from build123d import *

# Parameters (mm, degrees)
F0_W     = 73
F0_H     = 48
F1_DEPTH = 4
F0_W_2   = 79
F0_H_2   = 54
F2_DEPTH = 25
F3_W     = 2
F3_H     = 12
F4_DEPTH = 54
F5_W     = 20
F5_H     = 12
F6_DEPTH = 8
F7_W     = 3.5
F7_H     = 8
F8_DEPTH = 80
F9_R     = 3
F10_R    = 1


with BuildPart() as f1:
    # F0 (on Top) → F1 (new body)
    with BuildSketch(Plane.XY):
        Rectangle(F0_W, F0_H)
    extrude(amount=F1_DEPTH)

    # F0 (on Top) → F2 (join)
    with BuildSketch(Plane.XY):
        Rectangle(F0_W_2, F0_H_2)
        Rectangle(F0_W, F0_H, mode=Mode.SUBTRACT)
    extrude(amount=F2_DEPTH)

    # F3 (on face) → F4 (join)
    with BuildSketch(Plane.XZ.offset(27)):
        with Locations((40.5, 19)):
            Rectangle(F3_W, F3_H)
        Polygon((39.5, 13), (39.5, 0), (41.5, 13), align=None)
        with Locations((-40.5, 19)):
            Rectangle(F3_W, F3_H)
        Polygon((-41.5, 13), (-39.5, 0), (-39.5, 13), align=None)
    extrude(amount=-F4_DEPTH)

    # F5 (on face) → F6 (join)
    with BuildSketch(Plane(origin=(0, 27, 0), x_dir=(-1, 0, 0), z_dir=(0, 1, 0))):
        with Locations((-25.5, 19)):
            Rectangle(F5_W, F5_H)
        with Locations((25.5, 19)):
            Rectangle(F5_W, F5_H)
    extrude(amount=F6_DEPTH)

    # F7 (on face) → F8 (cut)
    with BuildSketch(Plane(origin=(-35.5, 0, 0), x_dir=(0, -1, 0), z_dir=(-1, 0, 0))):
        with Locations((-28.75, 17)):
            Rectangle(F7_W, F7_H)
    extrude(amount=-F8_DEPTH, mode=Mode.SUBTRACT)

    # F9
    f9_edges = [f1.edges().sort_by_distance(p)[0] for p in [
        (0, -24, 4),
        (36.5, 0, 4),
        (0, 24, 4),
        (-36.5, 0, 4),
    ]]
    fillet(f9_edges, radius=F9_R)

    # F10
    f10_edges = [f1.edges().sort_by_distance(p)[0] for p in [
        (0, -27, 25),
        (41.5, 0, 25),
        (38.5, 27, 25),
        (35.5, 31, 25),
        (25.5, 35, 25),
        (15.5, 31, 25),
        (0, 27, 25),
        (-15.5, 31, 25),
        (-25.5, 35, 25),
        (-35.5, 31, 25),
        (-38.5, 27, 25),
        (-41.5, 0, 25),
        (36.5, 0, 25),
        (0, -24, 25),
        (-36.5, 0, 25),
        (0, 24, 25),
        (0, -27, 0),
        (39.5, 0, 0),
        (0, 27, 0),
        (-39.5, 0, 0),
        (-40.5, -27, 6.5),
        (-41.5, -27, 19),
        (41.5, -27, 19),
        (40.5, -27, 6.5),
        (41.5, 0, 13),
        (40.5, 27, 6.5),
        (41.5, 27, 19),
        (-41.5, 0, 13),
        (-40.5, 27, 6.5),
        (-41.5, 27, 19),
        (-15.5, 35, 19),
        (-25.5, 35, 13),
        (-35.5, 35, 19),
        (35.5, 35, 19),
        (25.5, 35, 13),
        (15.5, 35, 19),
        (25.5, 30.5, 13),
        (15.5, 32.75, 13),
        (35.5, 32.75, 13),
        (-25.5, 30.5, 13),
        (-35.5, 32.75, 13),
        (-15.5, 32.75, 13),
        (-15.5, 27, 23),
        (-15.5, 28.75, 21),
        (-15.5, 30.5, 17),
        (35.5, 27, 23),
        (35.5, 28.75, 21),
        (35.5, 30.5, 17),
        (15.5, 30.5, 17),
        (15.5, 28.75, 21),
        (15.5, 27, 23),
        (-35.5, 30.5, 17),
        (-35.5, 28.75, 21),
        (-35.5, 27, 23),
        (25.5, 27, 21),
        (-25.5, 27, 21),
    ]]
    fillet(f10_edges, radius=F10_R)


solid = f1.part
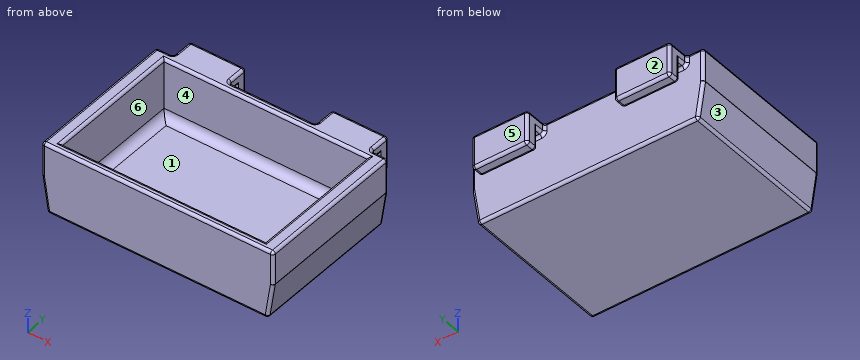
Geometry check sheet. Reference: the model listing, model coordinates, mm. Face numbers are marked on the shaded views. A direction names the side the tool comes from. Give positions to 0.01 mm unless a question says otherwise; leave off trailing zeros. Order: outer loops, then holes, each group sorted by start corner. A loop starts at its lowest first (then second) coordinate and runs counter-clockwise, first axis right, second up.
1) Gauge pin test, flat ends, axial feed: pin 1 (3 mm diameter, centred on y = 32, z = 20, fed in from +X); pin 2 (3 mm diameter, centred on x = -29, y = 29.5, fed in from -Z); pin 3 (5 mm diameter, centred on y = 32, z = 18, fed in from -X). Record the tip position at first contact, or that the pin passes through.
Results are:
pin 1: stops at x = 35.5
pin 2: stops at z = 13.13
pin 3: stops at x = -35.5
2) Cross-section at A-A (z = 17.25). Record the boundary of the cut face in (x, y).
Results are:
outline: (-41.5, -26) arc R1 ccw to (-40.5, -27) - (40.5, -27) arc R1 ccw to (41.5, -26) - (41.5, 26) arc R1 ccw to (40.5, 27) - (-40.5, 27) arc R1 ccw to (-41.5, 26) - close; (-35.5, 31.5) arc R1 ccw to (-34.5, 30.5) - (-16.5, 30.5) arc R1 ccw to (-15.5, 31.5) - (-15.5, 34) arc R1 ccw to (-16.5, 35) - (-34.5, 35) arc R1 ccw to (-35.5, 34) - close; (15.5, 31.5) arc R1 ccw to (16.5, 30.5) - (34.5, 30.5) arc R1 ccw to (35.5, 31.5) - (35.5, 34) arc R1 ccw to (34.5, 35) - (16.5, 35) arc R1 ccw to (15.5, 34) - close; hole (-36.5, -24) - (36.5, -24) - (36.5, 24) - (-36.5, 24) - close
3) Draft check along X on the marked faces 1, 2, 3 and 4. Enter one of: released by +X, released by -X, zero draft, split by the parting line, or undercut.
Results are:
face 1: undercut
face 2: zero draft
face 3: released by -X
face 4: undercut
4) Material ranges on probe 1 along Y at (x, z) = (-34.5, 17); probe 2 along Y at (x, z) = (36, 11.5); probe 3 along Z at (x, y) = (-6, 21), recorded low to high.
Results are:
probe 1: y = -27 to -24, 24 to 27, 30.5 to 35
probe 2: y = -27 to -24, 24 to 27
probe 3: z = 0 to 4
5) Cross-section at B-B (z = 23). Record the boundary of the cut face in (x, y).
Results are:
outline: (-41.5, -26) arc R1 ccw to (-40.5, -27) - (40.5, -27) arc R1 ccw to (41.5, -26) - (41.5, 26) arc R1 ccw to (40.5, 27) - (36.5, 27) arc R1 cw to (35.5, 28) - (35.5, 34) arc R1 ccw to (34.5, 35) - (16.5, 35) arc R1 ccw to (15.5, 34) - (15.5, 28) arc R1 cw to (14.5, 27) - (-14.5, 27) arc R1 cw to (-15.5, 28) - (-15.5, 34) arc R1 ccw to (-16.5, 35) - (-34.5, 35) arc R1 ccw to (-35.5, 34) - (-35.5, 28) arc R1 cw to (-36.5, 27) - (-40.5, 27) arc R1 ccw to (-41.5, 26) - close; hole (-36.5, -24) - (36.5, -24) - (36.5, 24) - (-36.5, 24) - close
6) Cross-section at D-D (y = -19.5). Record the boundary of the cut face in (x, z).
Results are:
outline: (-41.5, 13.08) arc R1 ccw to (-41.49, 12.92) - (-39.63, 0.85) arc R1 ccw to (-38.64, 0) - (38.64, 0) arc R1 ccw to (39.63, 0.85) - (41.49, 12.92) arc R1 ccw to (41.5, 13.08) - (41.5, 24) arc R1 ccw to (40.5, 25) - (37.5, 25) arc R1 ccw to (36.5, 24) - (36.5, 7) arc R3 cw to (33.5, 4) - (-33.5, 4) arc R3 cw to (-36.5, 7) - (-36.5, 24) arc R1 ccw to (-37.5, 25) - (-40.5, 25) arc R1 ccw to (-41.5, 24) - close
7) Cross-section at C-C (x = -4). Record the boundary of the cut face in (y, z), then the cut area to 3 significant figures.
Results are:
outline: (-27, 1) arc R1 ccw to (-26, 0) - (26, 0) arc R1 ccw to (27, 1) - (27, 24) arc R1 ccw to (26, 25) - (25, 25) arc R1 ccw to (24, 24) - (24, 7) arc R3 cw to (21, 4) - (-21, 4) arc R3 cw to (-24, 7) - (-24, 24) arc R1 ccw to (-25, 25) - (-26, 25) arc R1 ccw to (-27, 24) - close
area: 345 mm2
8) Tool access check on the marked faces 5 and 6. Record the directions out of +Z, -Z, +X, -X, +Y, -Y that give a thin tool (end or side, any length) a straight path to the whole face; none if there is none.
Results are:
face 5: +Z, -Z, +X, -X, +Y
face 6: +Z
